Check sheet for the modelled part. Datum: model origin and axes. Units: mm. A direction names the side the tool comes from. Round coordinates to 2 decimals unless told otherwise and drop trailing zeros. Order: outer loops, then holes, each group sorted by start corner. A loop starts at its lowest first (then second) coordinate and runs counter-clockwise, first axis right, second up.
(1) Sectioned sample at B-B, the plane x = 48. Enter the section's corners in (y, z).
(2) Thickness scan on probe 1 along Y at (x, z) = (50, 8.5); probe 2 along X at (y, z) = (-2, 3); probe 3 along Z at (x, y) = (0, 8). Record the ranges inside material, lowest first.
(3) Sectioned sample at A-A, the plane z = 2.75. Enter the section's corners in (x, y).
(4) Mould release check, pull along Y, two halves, no side actions. Record for faces 4 (the flat face through (-1.4, 3.05, 4.8)), 5 (the flat face through (5, 15, 6)), 6 (the flat face through (21, 0, 12.7)): released by +Y, released by -Y, zero draft, split by the parting line, or undercut.
(5) Sectioned sample at D-D, the plane z = 6.35. Enter the section's corners in (x, y), and give its area (3 significant figures).
(6) Depth check by flat-ended pin: pin 1 (2 mm diameter, centred on y = 7, z = 3, fed in from -X); pin 2 (5 mm diameter, centred on y = 8, z = 9.5, fed in from -X); pin 3 (1.5 mm diameter, centred on x = 16.5, z = 5.5, fed in from -Y). Enter the tip coordinate at first touch or a pass-through.
(7) Sectioned sample at C-C, the plane y = 1. Enter the section's corners in (x, z).
(8) Tool access check on faces 1 (the flat face through (0, -3.05, 6)), 2 (the cylindrical face through (58.74, -0.2, 6.26)), 3 (the cylindrical face through (-0.632, 8.941, 4.826)). Record the directions out of +Z, -Z, +X, -X, +Y, -Y that give a thin tool (end or side, any length) a straight path to the whole face; none if there is none.
```python
from build123d import *

# Parameters (mm, degrees)
SKETCH1_W                       = 6.1
SKETCH1_H                       = 6.1
BOSS_EXTRUDE1_DEPTH             = 12.7
TAP_DRILL_FOR_M4X0_7_TAP1_D     = 3.3
TAP_DRILL_FOR_M4X0_7_TAP1_DEPTH = 11.95
M5_CLEARANCE_HOLE1_D            = 5.3
FILLET1_R                       = 5


with BuildPart() as part:
    # Sketch1 → Boss-Extrude1 (new body)
    with BuildSketch(Plane.XY):
        with BuildLine():
            Line((50, 9.920327772), (10, 15))
            Line((10, 15), (0, 15))
            ThreePointArc((0, 15), (-15, 0), (0, -15))
            Line((0, -15), (10, -15))
            Line((10, -15), (50, -9.920327772))
            ThreePointArc((50, -9.920327772), (58.740199663, 0), (50, 9.920327772))
        make_face()
        Rectangle(SKETCH1_W, SKETCH1_H, mode=Mode.SUBTRACT)
    extrude(amount=BOSS_EXTRUDE1_DEPTH)

    # Tap Drill for M4x0.7 Tap1
    with Locations(Plane(origin=(0, 15, 6.35), x_dir=(0, 0, 1), z_dir=(0, 1, 0))):
        with Locations((0, 0)):
            Hole(TAP_DRILL_FOR_M4X0_7_TAP1_D / 2, depth=TAP_DRILL_FOR_M4X0_7_TAP1_DEPTH)

    # M5 Clearance Hole1 (through all)
    with Locations(Plane(origin=(50, 0, 0), x_dir=(-1, 0, 0), z_dir=(0, 0, -1))):
        with Locations((0, 0)):
            Hole(M5_CLEARANCE_HOLE1_D / 2)

    # Fillet1
    fillet1_edges = [part.edges().sort_by_distance(p)[0] for p in [
        (10, 15, 6.35),
        (10, -15, 6.35),
    ]]
    fillet(fillet1_edges, radius=FILLET1_R)


solid = part.part
```
Derived:
1. outline: (-10.17, 0) - (-1.74, 0) - (-1.74, 12.7) - (-10.17, 12.7) - close; (1.74, 0) - (10.17, 0) - (10.17, 12.7) - (1.74, 12.7) - close
2. probe 1: y = -9.92 to -2.65, 2.65 to 9.92
2. probe 2: x = -14.87 to -3.05, 3.05 to 48.26, 51.74 to 58.54
2. probe 3: z = 0 to 4.7, 8 to 12.7
3. outline: (0, -15) - (9.68, -15) arc R5 ccw to (10.31, -14.96) - (50, -9.92) arc R10 ccw to (50, 9.92) - (10.31, 14.96) arc R5 ccw to (9.68, 15) - (0, 15) arc R15 ccw to start; hole (-3.05, -3.05) - (3.05, -3.05) - (3.05, 3.05) - (-3.05, 3.05) - close; hole circle Ø5.3 at (50, 0)
4. face 4: undercut
4. face 5: released by +Y
4. face 6: zero draft
5. outline: (-3.05, -3.05) - (-3.05, 3.05) - (-1.65, 3.05) - (-1.65, 14.91) arc R15 ccw to (0, -15) - (9.68, -15) arc R5 ccw to (10.31, -14.96) - (50, -9.92) arc R10 ccw to (50, 9.92) - (10.31, 14.96) arc R5 ccw to (9.68, 15) - (1.65, 15) - (1.65, 3.05) - (3.05, 3.05) - (3.05, -3.05) - close; hole circle Ø5.3 at (50, 0)
5. area: 1,680 mm2
6. pin 1: stops at x = -13.75
6. pin 2: stops at x = -13.96
6. pin 3: stops at y = -14.27
7. outline: (-14.97, 0) - (-3.05, 0) - (-3.05, 12.7) - (-14.97, 12.7) - close; (3.05, 0) - (47.55, 0) - (47.55, 12.7) - (3.05, 12.7) - close; (52.45, 0) - (58.69, 0) - (58.69, 12.7) - (52.45, 12.7) - close
8. face 1: +Z, -Z
8. face 2: +Z, -Z, +X
8. face 3: +Y
